```python
from build123d import *

# Parameters (mm, degrees)
F0_W      = 32
F0_H      = 36
F1_DEPTH  = 2.5
F3_DEPTH  = 180
F4_R      = 1
F5_R      = 2
F6_R      = 3
F7_DEPTH  = 5
F9_R      = 3
F9_R_2    = 2.25
F10_DEPTH = 1
F11_SIZE  = 3
F12_SIZE  = 4


with BuildPart() as f1:
    # F0 (on Top) → F1 (new body)
    with BuildSketch(Plane.XY):
        with Locations((0, 1)):
            Rectangle(F0_W, F0_H)
    extrude(amount=-F1_DEPTH)

    # F2 (on face) → F3 (join)
    with BuildSketch(Plane.XY):
        Polygon((12.5, -12.5), (12.5, 12.5), (-12.5, 12.5), (-12.5, -12.5), (-7.5, -12.5), (-7.5, -11.5), (-11.5, -11.5), (-11.5, 11.5), (11.5, 11.5), (11.5, -11.5), (7.5, -11.5), (7.5, -12.5), align=None)
    extrude(amount=F3_DEPTH)

    # F4
    f4_edges = [f1.edges().sort_by_distance(p)[0] for p in [
        (-11.5, 11.5, 90),
        (11.5, 11.5, 90),
        (-11.5, -11.5, 90),
        (11.5, -11.5, 90),
    ]]
    fillet(f4_edges, radius=F4_R)

    # F5
    f5_edges = [f1.edges().sort_by_distance(p)[0] for p in [
        (-12.5, 12.5, 90),
        (12.5, 12.5, 90),
        (12.5, -12.5, 90),
        (-12.5, -12.5, 90),
    ]]
    fillet(f5_edges, radius=F5_R)

    # F6 (on face) → F7 (join)
    with BuildSketch(Plane.XZ.offset(-11.5)):
        with Locations((0, 5)):
            Circle(F6_R)
    extrude(amount=F7_DEPTH)

    # F9 (on offset) → F10 (cut, symmetric)
    with BuildSketch(Plane.XZ.offset(-8.5)):
        with Locations((0, 5)):
            Circle(F9_R)
        with Locations((0, 5)):
            Circle(F9_R_2, mode=Mode.SUBTRACT)
    extrude(amount=F10_DEPTH, both=True, mode=Mode.SUBTRACT)

    # F11
    f11_edges = [f1.edges().sort_by_distance(p)[0] for p in [
        (-16, -17, -1.25),
        (16, -17, -1.25),
    ]]
    chamfer(f11_edges, length=F11_SIZE)

    # F12
    f12_edges = [f1.edges().sort_by_distance(p)[0] for p in [
        (16, 19, -1.25),
        (-16, 19, -1.25),
    ]]
    chamfer(f12_edges, length=F12_SIZE)


solid = f1.part
```
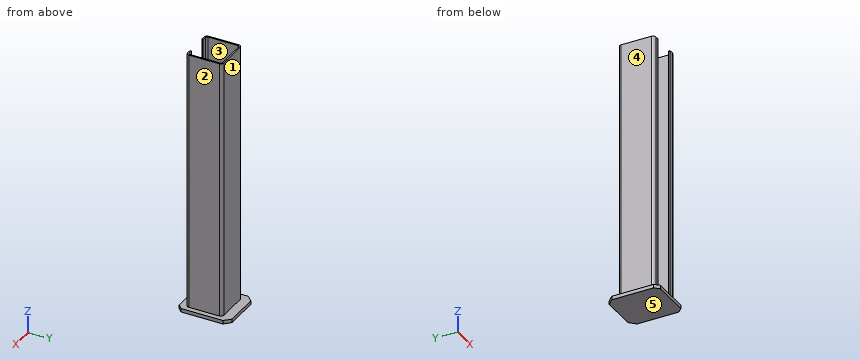
Work out the finished part from the listing and answer in its coordinate system (mm). Face numbers are marked on the shaded views. A direction names the side the tool comes from. Give positions to 0.01 mm unless a question says otherwise; leave off trailing zeros. Order: outer loops, then holes, each group sorted by start corner. A loop starts at its lowest first (then second) coordinate and runs counter-clockwise, first axis right, second up. Notation, with made-up numbers: (-7.5, 63.25) -> (13.5, 63.25) arc R26 cw to (13.5, 93.25) -> close; hole circle Ø9 at (38.25, 14). An arc over 180 degrees is marked (long way). Answer as CSV lines item,"result". Start each with the question number.
(1) Section C-C, the plane y = -5.5 is taken. Write down the section's boundary in (x, z).
(2) For a pull along Y with two mould halves and no side action, classify the marked faces 1, 2 and 3 as released by +Y, released by -Y, zero draft, split by the parting line, or undercut.
(3) Each of these flat-tipped pins is pushed along its axis until it touches: pin 1 Ø17 at (y, z) = (-4.5, 68.5) entering from -X; pin 2 Ø5 at (y, z) = (-12, 153) entering from +X; pin 3 Ø2.5 at (x, z) = (-8.5, 114) entering from -Y. Where does it stop, or does it pass through?
(4) Consider line 1 along X through (y, z) = (-10.5, 69); line 2 along Z through (x, y) = (0.5, 0.5). Determine where each line is inside the solid, lowest interval first.
(5) Which of the six approach directions +Z, -Z, +X, -X, +Y, -Y give full straight-line access (tool end or side, diameter ignored) to the marked faces 4 and 5?
(6) Section B-B, the plane x = 0 is taken. Write down the section's boundary in (y, z), plus the area to 3 significant figures.
(7) Section D-D, the plane z = 62 is taken. Write down the section's boundary in (x, y).
Entries:
1,outline,"(-16, -2.5) -> (16, -2.5) -> (16, 0) -> (12.5, 0) -> (12.5, 180) -> (11.5, 180) -> (11.5, 0) -> (-11.5, 0) -> (-11.5, 180) -> (-12.5, 180) -> (-12.5, 0) -> (-16, 0) -> close"
2,face 1,"released by +Y"
2,face 2,"zero draft"
2,face 3,"undercut"
3,pin 1,"x = -12.5"
3,pin 2,"x = 12.5"
3,pin 3,"y = -12.5"
4,line 1,"-12.5 to -11.5, 11.5 to 12.5"
4,line 2,"-2.5 to 0"
5,face 4,"+Z, -X, +Y, -Y"
5,face 5,"-Z, +X, -X, +Y, -Y"
6,outline,"(-17, -2.5) -> (19, -2.5) -> (19, 0) -> (12.5, 0) -> (12.5, 180) -> (11.5, 180) -> (11.5, 8) -> (9.5, 8) -> (9.5, 7.25) -> (7.5, 7.25) -> (7.5, 8) -> (6.5, 8) -> (6.5, 2) -> (7.5, 2) -> (7.5, 2.75) -> (9.5, 2.75) -> (9.5, 2) -> (11.5, 2) -> (11.5, 0) -> (-17, 0) -> close"
6,area,"297 mm²"
7,outline,"(-12.5, -10.5) arc R2 ccw to (-10.5, -12.5) -> (-7.5, -12.5) -> (-7.5, -11.5) -> (-10.5, -11.5) arc R1 cw to (-11.5, -10.5) -> (-11.5, 10.5) arc R1 cw to (-10.5, 11.5) -> (10.5, 11.5) arc R1 cw to (11.5, 10.5) -> (11.5, -10.5) arc R1 cw to (10.5, -11.5) -> (7.5, -11.5) -> (7.5, -12.5) -> (10.5, -12.5) arc R2 ccw to (12.5, -10.5) -> (12.5, 10.5) arc R2 ccw to (10.5, 12.5) -> (-10.5, 12.5) arc R2 ccw to (-12.5, 10.5) -> close"
